The listing builds one solid part. Answer for the finished solid, in the listing's coordinates (mm). A direction names the side the tool comes from. Coordinates: 2 decimals unless noted, no trailing zeros. Order: outer loops, then holes, each group sorted by start corner. A loop starts at its lowest first (then second) coordinate and runs counter-clockwise, first axis right, second up. Notation, with made-up numbers: (-17.5, -24) -> (9.5, -24) arc R12 cw to (9.5, -4) -> close; hole circle Ø10 at (46.5, -29). An arc over 180 degrees is marked (long way). Write item = value, one per line.
from build123d import *

# Parameters (mm, degrees)
BOSS_EXTRUDE1_DEPTH = 457.2
SKETCH3_W           = 2.54
SKETCH3_H           = 2.032


with BuildPart() as part:
    # Sketch1 → Boss-Extrude1 (new body)
    with BuildSketch(Plane(origin=(0, 0, 0), x_dir=(1, 0, 0), z_dir=(0, 1, 0))):
        Polygon((7.332348419, 0), (3.666174209, 6.35), (-3.666174209, 6.35), (-7.332348419, 0), (-3.666174209, -6.35), (3.666174209, -6.35), align=None)
        Polygon((1.443375673, 2.5), (-1.443375673, 2.5), (-2.886751346, 0), (-1.443375673, -2.5), (1.443375673, -2.5), (2.886751346, 0), align=None, mode=Mode.SUBTRACT)
    extrude(amount=BOSS_EXTRUDE1_DEPTH)

    # Sketch3 → Cut-Revolve2 (revolve, cut)
    with BuildSketch(Plane(origin=(0, 0, 0), x_dir=(0, 0, -1), z_dir=(1, 0, 0)), mode=Mode.PRIVATE) as cut_revolve2_sk:
        with Locations((6.2865, 55.499)):
            Rectangle(SKETCH3_W, SKETCH3_H)
        with Locations((6.2865, 5.207)):
            Rectangle(SKETCH3_W, SKETCH3_H)
    revolve(cut_revolve2_sk.sketch.rotate(Axis((0, 457.2, 0), (0, -1, 0)), 180), axis=Axis((0, 457.2, 0), (0, -1, 0)), mode=Mode.SUBTRACT)


solid = part.part
Q1. Find the intervals of material crossed by line 1 along Y through (x, z) = (3.5, 4.75) (3 decimals); line 2 along Z through (x, y) = (1.25, 286); line 3 along Z through (x, y) = (2.5, 209), in increasing order.
The answers:
line_1 = 0 to 4.191, 6.223 to 54.483, 56.515 to 457.2
line_2 = -6.35 to -2.5, 2.5 to 6.35
line_3 = -6.35 to -0.67, 0.67 to 6.35
Q2. Each of these flat-tipped pins is pushed along its axis until it touches: pin 1 Ø1.5 at (y, z) = (94, -1) entering from -X; pin 2 Ø1.5 at (y, z) = (164, -2) entering from +X. Where does it stop, or does it pass through?
The answers:
pin_1 = -7.19
pin_2 = 6.61
Q3. The mould has two halves that part along Y. Classify faces 3 (the face through (0, 30, -6.35)), 4 (the face through (3.2, 0, -0.1)), 5 (the face through (-2, 54.483, 5)), 6 (the face through (3.2, 457.2, -0.1)): released by +Y, released by -Y, zero draft, split by the parting line, or undercut.
The answers:
face_3 = zero draft
face_4 = released by -Y
face_5 = undercut
face_6 = released by +Y
Q4. A tool of negligible diameter and unlimited length cuts with its end or side. For faces 1 (the face through (-2, 6.223, 5)), 2 (the face through (0, 254, 6.35)), from which of +Z, -Z, +X, -X, +Y, -Y can it reach the whole face along a straight path? Write none if from no direction.
The answers:
face_1 = none
face_2 = +Z, +X, -X, +Y, -Y
Q5. Section A-A, the plane y = 334 is taken. Give the vertices of the cut face in (x, z).
The answers:
outline = (-7.33, 0) -> (-3.67, -6.35) -> (3.67, -6.35) -> (7.33, 0) -> (3.67, 6.35) -> (-3.67, 6.35) -> close; hole (-2.89, 0) -> (-1.44, -2.5) -> (1.44, -2.5) -> (2.89, 0) -> (1.44, 2.5) -> (-1.44, 2.5) -> close
